Read the model definition and answer for the solid it produces. Units are mm, in the model's axes. Face numbers are marked on the shaded views. Coordinates: 2 decimals unless noted, no trailing zeros. Write each loop counter-clockwise with the first axis right and the second up, starting at its lowest first coordinate (ties: lowest second). Pieces come first, ordered by that corner, then holes. Notation, with made-up numbers: (21.5, -20.5) -> (70.5, -20.5) arc R9 ccw to (70.5, -15.5) -> close; hole circle Ø10 at (77.25, 67). An arc over 180 degrees is marked (long way). One line per item, written item: value. Start each with the question number.
Autodesk Inventor part; units mm, degrees
ref_plane "YZ Plane" through (0, 0, 0) normal (1, 0, 0) x (0, 1, 0)
ref_plane "XZ Plane" through (0, 0, 0) normal (0, 1, 0) x (-1, 0, 0)
ref_plane "XY Plane" through (0, 0, 0) normal (0, 0, 1) x (1, 0, 0)
sketch "Sketch1" plane through (0, 0, 0) normal (0, 1, 0) x (-1, 0, 0)
  line L0 (-27.75, 43.375) -> (27.75, 43.375)
  line L1 (27.75, 43.375) -> (27.75, -43.375)
  line L2 (27.75, -43.375) -> (-27.75, -43.375)
  line L3 (-27.75, -43.375) -> (-27.75, 43.375)
  line L4 (-27.75, 43.375) -> (27.75, -43.375) construction
  line L5 (27.75, 43.375) -> (-27.75, -43.375) construction
  point P0 (0, 0)
  dimension "d0" = 86.75
  dimension "d1" = 55.5
extrude "Extrusion1" add sketch "Sketch1" along normal blind 8
sketch "Sketch2" plane through (0, 8, 0) normal (0, 1, 0) x (1, 0, 0)
  line L0 (25.75, -41.375) -> (-25.75, -41.375)
  line L1 (-25.75, -41.375) -> (-25.75, 41.375)
  line L2 (-25.75, 41.375) -> (25.75, 41.375)
  line L3 (25.75, 41.375) -> (25.75, -41.375)
  line L4 (25.75, -41.375) -> (-25.75, 41.375) construction
  line L5 (-25.75, -41.375) -> (25.75, 41.375) construction
  point P0 (0, 0)
  dimension "d4" = 51.5
  dimension "d5" = 82.75
extrude "Extrusion2" cut sketch "Sketch2" against normal blind 2
sketch "Sketch3" plane through (0, 6, 0) normal (0, 1, 0) x (1, 0, 0)
  line L0 (24.25, 39.875) -> (-24.25, 39.875)
  line L1 (-24.25, 39.875) -> (-24.25, -39.875)
  line L2 (-24.25, -39.875) -> (24.25, -39.875)
  line L3 (24.25, -39.875) -> (24.25, 39.875)
  line L4 (24.25, 39.875) -> (-24.25, -39.875) construction
  line L5 (-24.25, 39.875) -> (24.25, -39.875) construction
  point P0 (0, 0)
  dimension "d8" = 79.75
  dimension "d9" = 48.5
extrude "Extrusion3" cut sketch "Sketch3" against normal blind 4
sketch "Sketch4" plane through (0, 2, 0) normal (0, 1, 0) x (1, 0, 0)
  circle A0 centre (0, -37.375) radius 4.5
  circle A1 centre (0, 37.375) radius 4.5
  line L0 (24.25, -39.875) -> (-24.25, -39.875)
  line L1 (25.75, -41.375) -> (-25.75, -41.375)
  circle A2 centre (0, -37.375) radius 1.5
  circle A3 centre (0, 37.375) radius 1.5
  point P0 (0, 0)
  point P1 (-3.7417, -39.875)
  point P2 (3.7417, -39.875)
  dimension "d12" = 9
  dimension "d13" = 9
  dimension "d14" = 74.75
  dimension "d16" = 4
  dimension "d17" = 3
  dimension "d18" = 3
extrude "Extrusion4" add sketch "Sketch4" along normal blind 4 contours A0 L0 | A1
sketch "Sketch5" plane through (27.75, 0, 43.375) normal (1, 0, 0) x (0, 0, -1)
  line L0 (84.75, 8) -> (2, 8)
  line L1 (0, 0) -> (86.75, 0)
  line L2 (34.375, 8) -> (52.375, 8)
  line L3 (52.375, 8) -> (52.375, 0)
  line L4 (52.375, 0) -> (34.375, 0)
  line L5 (34.375, 0) -> (34.375, 8)
  point P0 (43.375, 0)
  point P1 (34.375, 4)
  point P2 (43.375, 0)
  point P3 (34.375, 0)
  point P4 (52.375, 8)
  dimension "d21" = 18
  dimension "d22" = 9
extrude "Extrusion5" add sketch "Sketch5" along normal blind 18
sketch "Sketch6" plane through (0, 8, 0) normal (0, 1, 0) x (1, 0, 0)
  line L0 (27.75, -43.375) -> (27.75, -9)
  line L1 (27.75, -9) -> (45.75, -9)
  point P0 (0, 0)
  point P1 (36.75, 0)
  dimension "d32" = 9
  dimension "d33" = 9
hole "Hole1" at (36.75, 8, 0) direction (0, -1, 0) diameter 7.1437 end through all counterbore diameter 11.1125 counterbore depth 6.35
fillet "Fillet2" radius 5 4 edges at (27.75, 4, 9) (45.75, 4, 9) (45.75, 4, -9) (27.75, 4, -9)
fillet "Fillet3" radius 2 4 edges at (27.75, 4, 43.375) (27.75, 4, -43.375) (-27.75, 4, -43.375) (-27.75, 4, 43.375)
properties part number "PermaProtoBase_HalfSizeScrewMount"
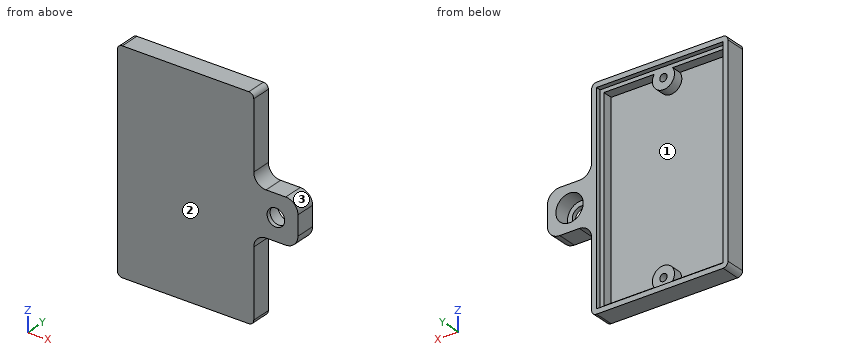
1. A cutting plane is placed at B-B on z = 0. Give the vertices of the cut face in (x, y).
2. A cutting plane is placed at C-C on x = -14.5. Give the vertices of the cut face in (y, z) (3 decimals), then the cut area to 4 significant figures.
3. For a pull along Z with two mould halves and no side action, classify the marked faces 1, 2 and 3 as +Z half, -Z half, draft (parallel to the pull), parting line (faces both ways), or undercut.
4. Given pin 1 (2.5 mm diameter, centred on y = 5.5, z = -26, fed in from +X); pin 2 (3 mm diameter, centred on y = 3.5, z = 11.5, fed in from +X); pin 3 (2.5 mm diameter, centred on x = 0, z = -37.375, fed in from +Y), each flat-ended and moving along its own axis, determine where each tip first touches the part or whether it passes through.
5. A cutting plane is placed at A-A on x = 36.75. Give the vertices of the cut face in (y, z), then the cut area to 3 significant figures.
6. Find the intervals of material crossed by probe 1 along Z at (x, y) = (0, 3.1) (3 decimals); probe 2 along X at (y, z) = (2.75, 20.5); probe 3 along X at (y, z) = (7.25, 20), in increasing order. Write a range as from..to.
7. A cutting plane is placed at D-D on y = 3.75. Count the separate pieces of the cut face and the enclosed holes in it, then the cut area to 3 significant figures.
Derived:
1. outline: (-27.75, 0) -> (33.18, 0) -> (33.18, 1.65) -> (31.19, 1.65) -> (31.19, 8) -> (25.75, 8) -> (25.75, 6) -> (24.25, 6) -> (24.25, 2) -> (-24.25, 2) -> (-24.25, 6) -> (-25.75, 6) -> (-25.75, 8) -> (-27.75, 8) -> close; (40.32, 0) -> (45.75, 0) -> (45.75, 8) -> (42.31, 8) -> (42.31, 1.65) -> (40.32, 1.65) -> close
2. outline: (0, -43.375) -> (8, -43.375) -> (8, -41.375) -> (6, -41.375) -> (6, -39.875) -> (2, -39.875) -> (2, 39.875) -> (6, 39.875) -> (6, 41.375) -> (8, 41.375) -> (8, 43.375) -> (0, 43.375) -> close
2. area: 209.5 mm2
3. face 1: undercut
3. face 2: draft
3. face 3: +Z half
4. pin 1: stops at x = 27.75
4. pin 2: stops at x = 29.75
4. pin 3: stops at y = 2
5. outline: (0, -9) -> (8, -9) -> (8, -5.56) -> (1.65, -5.56) -> (1.65, -3.57) -> (0, -3.57) -> close; (0, 3.57) -> (1.65, 3.57) -> (1.65, 5.56) -> (8, 5.56) -> (8, 9) -> (0, 9) -> close
5. area: 61.6 mm2
6. probe 1: z = -43.375..-38.875, -35.875..-32.875, 32.875..35.875, 38.875..43.375
6. probe 2: x = -27.75..-24.25, 24.25..27.75
6. probe 3: x = -27.75..-25.75, 25.75..27.75
7. separate pieces: 1
7. enclosed holes: 4
7. area: 1,260 mm2
